Design review of the part built by this model. Coordinates are the model's own, in mm. Face numbers are marked on the shaded views. A direction names the side the tool comes from. Round coordinates to 2 decimals unless told otherwise and drop trailing zeros. Write each loop counter-clockwise with the first axis right and the second up, starting at its lowest first coordinate (ties: lowest second). Pieces come first, ordered by that corner, then holes. Notation, with made-up numbers: (-33, -3.75) -> (-13, -3.75) arc R20 ccw to (-13, 29.25) -> close; hole circle Ø11 at (-12.5, 13.5). An arc over 180 degrees is marked (long way). One line per question, with ' | ' between items. Start each with the question number.
1) Consider section C-C (x = 8.5). Give the boundary of the cut face in (y, z).
2) Consider section A-A (z = 0). Give the boundary of the cut face in (x, y).
3) Mouldability with a two-part tool opening along X and no side actions: class the marked faces 3, 4 and 5 as +X half, -X half, draft (parallel to the pull), parting line (faces both ways), or undercut.
4) For the marked faces 1 and 2, list the 3-axis set-ups (+Z, -Z, +X, -X, +Y, -Y) from which the entire face can be reached by the end or side of a thin tool; tool diameter is ignored.
5) For probe 1 along X at (y, z) = (2, -3); probe 2 along Z at (x, y) = (1.6, 0); probe 3 along X at (y, z) = (0.75, -1), list the stretches that pass through material, from the lowest coordinate up.
6) Insertion check: pin 1 Ø2 at (x, y) = (1.5, -3.5) entering from +Z; pin 2 Ø2 at (x, y) = (5.5, 1.5) entering from -Z. Each pin has a flat end and moves straight along its axis. Give the tip position at first contact, or say it passes through.
7) Consider section D-D (x = 1.5). Give the boundary of the cut face in (y, z).
```python
from build123d import *

# Parameters (mm, degrees)
F2_SIZE  = 1
F3_R     = 3
F4_DEPTH = 3


with BuildPart() as f1:
    # F0 (on Front) → F1 (revolve)
    with BuildSketch(Plane.XZ):
        Polygon((3, 4.75), (0, 4.75), (0, 0), (9, 0), (9, 4.75), (6, 4.75), (6, 3.25), (3, 3.25), align=None)
    revolve(axis=Axis((4.5, 0, 0), (1, 0, 0)))

    # F2
    f2_edges = [f1.edges().sort_by_distance(p)[0] for p in [
        (0, 0, -4.75),
        (9, 0, -4.75),
    ]]
    chamfer(f2_edges, length=F2_SIZE)

    # F3 (on face) → F4 (cut)
    with BuildSketch(Plane(origin=(0, 0, 0), x_dir=(0, -1, 0), z_dir=(-1, 0, 0))):
        Circle(F3_R)
    extrude(amount=-F4_DEPTH, mode=Mode.SUBTRACT)


solid = f1.part
```
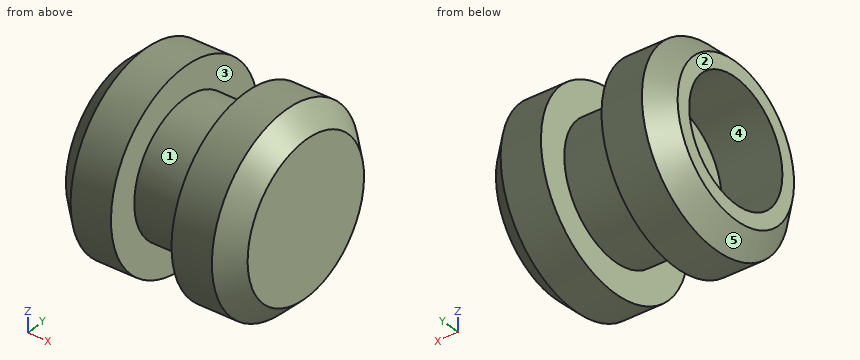
From the geometry:
1) outline: circle Ø8.5 at (0, 0)
2) outline: (0, -3.75) -> (1, -4.75) -> (3, -4.75) -> (3, -3.25) -> (6, -3.25) -> (6, -4.75) -> (8, -4.75) -> (9, -3.75) -> (9, 3.75) -> (8, 4.75) -> (6, 4.75) -> (6, 3.25) -> (3, 3.25) -> (3, 4.75) -> (1, 4.75) -> (0, 3.75) -> (0, 3) -> (3, 3) -> (3, -3) -> (0, -3) -> close
3) face 3: undercut | face 4: draft | face 5: -X half
4) face 1: none | face 2: +Z, -Z, -X, +Y, -Y
5) probe 1: x = 0 to 3, 6 to 9 | probe 2: z = -4.75 to -3, 3 to 4.75 | probe 3: x = 3 to 9
6) pin 1: stops at z = 4.04 | pin 2: stops at z = -4.71
7) outline: circle Ø9.5 at (0, 0); hole circle Ø6 at (0, 0)
